```python
from build123d import *

# Parameters (mm, degrees)
SKETCH1_R           = 3.441866939
SKETCH1_R_2         = 3.819680327
SKETCH1_R_3         = 3.478478145
SKETCH1_R_4         = 3.546045212
SKETCH1_R_5         = 2.15
SKETCH1_R_6         = 1.75
SKETCH1_R_7         = 1.6
SKETCH1_R_8         = 1.5
BOSS_EXTRUDE1_DEPTH = 4.8
SKETCH8_W           = 40.1
SKETCH8_H           = 40.1
CUT_EXTRUDE3_DEPTH  = 1.8


with BuildPart() as part:
    # Sketch1 → Boss-Extrude1 (new body)
    with BuildSketch(Plane(origin=(0, 0, 0), x_dir=(1, 0, 0), z_dir=(0, 1, 0))):
        with BuildLine():
            Line((245, 5), (245, 17.432639589))
            ThreePointArc((245, 17.432639589), (246.464466094, 20.968173495), (250, 22.432639589))
            Line((250, 22.432639589), (260, 22.432639589))
            ThreePointArc((260, 22.432639589), (263.535533906, 23.897105683), (265, 27.432639589))
            Line((265, 27.432639589), (265, 132))
            ThreePointArc((265, 132), (263.535533906, 135.535533906), (260, 137))
            Line((260, 137), (169.363043016, 137))
            ThreePointArc((169.363043016, 137), (166.534615891, 135.828427125), (165.363043016, 133))
            Line((165.363043016, 133), (165.363043016, 125))
            ThreePointArc((165.363043016, 125), (164.48436336, 122.878679656), (162.363043016, 122))
            Line((162.363043016, 122), (143.363043016, 122))
            ThreePointArc((143.363043016, 122), (141.241722673, 122.878679656), (140.363043016, 125))
            Line((140.363043016, 125), (140.363043016, 133))
            ThreePointArc((140.363043016, 133), (139.191470141, 135.828427125), (136.363043016, 137))
            Line((136.363043016, 137), (-21.419472962, 137))
            ThreePointArc((-21.419472962, 137), (-24.955006868, 135.535533906), (-26.419472962, 132))
            Line((-26.419472962, 132), (-26.419472962, 4))
            ThreePointArc((-26.419472962, 4), (-25.247900086, 1.171572875), (-22.419472962, 0))
            Line((-22.419472962, 0), (0, 0))
            Line((0, 0), (240, 0))
            ThreePointArc((240, 0), (243.535533906, 1.464466094), (245, 5))
        make_face()
        with Locations((10.923340914, 52.745575572)):
            Circle(SKETCH1_R, mode=Mode.SUBTRACT)
        with Locations((87.123340914, 52.745575572)):
            Circle(SKETCH1_R_2, mode=Mode.SUBTRACT)
        with Locations((10.923340914, 128.945575572)):
            Circle(SKETCH1_R_3, mode=Mode.SUBTRACT)
        with Locations((87.123340914, 128.945575572)):
            Circle(SKETCH1_R_4, mode=Mode.SUBTRACT)
        with Locations((251.055268843, 40.693078652)):
            Circle(SKETCH1_R_5, mode=Mode.SUBTRACT)
        with Locations((250.907128745, 118.650785042)):
            Circle(SKETCH1_R_5, mode=Mode.SUBTRACT)
        with Locations((-9.383394869, 57.477183604)):
            Circle(SKETCH1_R_5, mode=Mode.SUBTRACT)
        with Locations((232.6, 9)):
            Circle(SKETCH1_R_6, mode=Mode.SUBTRACT)
        with Locations((-10.109931835, 117.018747652)):
            Circle(SKETCH1_R_5, mode=Mode.SUBTRACT)
        with Locations((175.026105079, 21.135490335)):
            Circle(SKETCH1_R_6, mode=Mode.SUBTRACT)
        with Locations((234.82067073, 51.7688297)):
            Circle(SKETCH1_R_7, mode=Mode.SUBTRACT)
        with Locations((212.16387073, 51.7688297)):
            Circle(SKETCH1_R_7, mode=Mode.SUBTRACT)
        with Locations((101.612778703, 56.992933905)):
            Circle(SKETCH1_R_5, mode=Mode.SUBTRACT)
        with Locations((168.022600915, 55.959262506)):
            Circle(SKETCH1_R_5, mode=Mode.SUBTRACT)
        with Locations((171.2, 32)):
            Circle(SKETCH1_R_8, mode=Mode.SUBTRACT)
        with Locations((171.2, 9.902)):
            Circle(SKETCH1_R_8, mode=Mode.SUBTRACT)
        with Locations((118.5, 11.8)):
            Circle(SKETCH1_R_6, mode=Mode.SUBTRACT)
        with Locations((161.2, 9.902)):
            Circle(SKETCH1_R_8, mode=Mode.SUBTRACT)
        with Locations((161.2, 32)):
            Circle(SKETCH1_R_8, mode=Mode.SUBTRACT)
        with Locations((156.7, 113.6)):
            Circle(SKETCH1_R_6, mode=Mode.SUBTRACT)
        with Locations((84.495, 114.3284)):
            Circle(SKETCH1_R_8, mode=Mode.SUBTRACT)
        with Locations((84.495, 91.6716)):
            Circle(SKETCH1_R_8, mode=Mode.SUBTRACT)
        with Locations((70.3284, 77.505)):
            Circle(SKETCH1_R_8, mode=Mode.SUBTRACT)
        with Locations((47.6716, 77.505)):
            Circle(SKETCH1_R_8, mode=Mode.SUBTRACT)
        with Locations((47.6716, 128.495)):
            Circle(SKETCH1_R_8, mode=Mode.SUBTRACT)
        with Locations((70.3284, 128.495)):
            Circle(SKETCH1_R_8, mode=Mode.SUBTRACT)
        with Locations((33.505, 12.7216)):
            Circle(SKETCH1_R_8, mode=Mode.SUBTRACT)
        with Locations((33.505, 35.3784)):
            Circle(SKETCH1_R_8, mode=Mode.SUBTRACT)
        with Locations((70.3284, 49.545)):
            Circle(SKETCH1_R_8, mode=Mode.SUBTRACT)
        with Locations((47.6716, 49.545)):
            Circle(SKETCH1_R_8, mode=Mode.SUBTRACT)
        with Locations((3.9, 5.3556)):
            Circle(SKETCH1_R_8, mode=Mode.SUBTRACT)
        with Locations((8.472, 35.353)):
            Circle(SKETCH1_R_8, mode=Mode.SUBTRACT)
        with Locations((-21.541231751, 12.61861449)):
            Circle(SKETCH1_R_8, mode=Mode.SUBTRACT)
        with Locations((-21.541231751, 35.27541449)):
            Circle(SKETCH1_R_8, mode=Mode.SUBTRACT)
    extrude(amount=BOSS_EXTRUDE1_DEPTH)

    # Sketch8 → Cut-Extrude3 (cut)
    with BuildSketch(Plane(origin=(0, 4.8, 0), x_dir=(1, 0, 0), z_dir=(0, 1, 0))):
        with Locations((59, 103)):
            Rectangle(SKETCH8_W, SKETCH8_H)
    extrude(amount=-CUT_EXTRUDE3_DEPTH, mode=Mode.SUBTRACT)


solid = part.part
```
Source: CAD feature listing. Evaluate the final solid. Frame: model axes, mm. A direction names the side the tool comes from. Give positions to 0.01 mm unless a question says otherwise; leave off trailing zeros. Put each result on its own line as item: value. Start each with the question number.
1) Draft query along X for faces 3 (the face through (10.177, 2.366, -49.386)), 4 (the face through (246.4, 2.4, -20.9)), 5 (the face through (89.177, 2.366, -55.966)), 6 (the face through (117, 0, -69)). Return one class per face: released by +X, released by -X, zero draft, split by the parting line, or undercut.
2) Contact query for a flat-ended pin moving along its axis: P1, Ø5, axis at x = 8.472, z = -35.353, coming from the -Y side. Output: stop coordinate, or through.
3) Reachability of faces 1 (the face through (263.5, 2.37, -23.86)), 2 (the face through (59, 3, -103)) from +Z, -Z, +X, -X, +Y, -Y: full face, straight path, thin tool, end or side. Return the list, or none.
4) Cut plane A-A (y = 3.95). State how many separate pieces and enclosed holes the cut face has, then the cut area to 3 significant figures.
5) Material intervals for probe 1 along Z at (x, y) = (161.5, 3.65); probe 2 along X at (y, z) = (3.7, -78); probe 3 along X at (y, z) = (4.35, -54), sorted ascending.
Results are:
1. face 3: undercut
1. face 4: released by +X
1. face 5: undercut
1. face 6: zero draft
2. P1: stops at y = 0
3. face 1: +Z, +X, +Y, -Y
3. face 2: +Y
4. separate pieces: 1
4. enclosed holes: 35
4. area: 37,000 mm2
5. probe 1: z = -122 to -33.47, -30.53 to -11.37, -8.43 to 0
5. probe 2: x = -26.42 to 46.26, 49.09 to 68.91, 71.74 to 265
5. probe 3: x = -26.42 to 7.72, 14.13 to 83.52, 90.73 to 167.14, 168.91 to 265
